```python
from build123d import *

# Parameters (mm, degrees)
SKETCH1_W           = 80
SKETCH1_H           = 80
SKETCH1_R           = 25
BOSS_EXTRUDE1_DEPTH = 10
SKETCH3_W           = 80
SKETCH3_H           = 80
SKETCH3_R           = 25
BOSS_EXTRUDE2_DEPTH = 10
SKETCH4_R           = 25
SKETCH4_W           = 80
SKETCH4_H           = 80
BOSS_EXTRUDE3_DEPTH = 10


with BuildPart() as part:
    # Sketch1 → Boss-Extrude1 (new body)
    with BuildSketch(Plane(origin=(0, 0, 0), x_dir=(1, 0, 0), z_dir=(0, 1, 0))):
        with Locations((40, -40)):
            Rectangle(SKETCH1_W, SKETCH1_H)
        with Locations((40, -40)):
            Circle(SKETCH1_R, mode=Mode.SUBTRACT)
        with Locations((120, -40)):
            Rectangle(SKETCH1_W, SKETCH1_H)
        with Locations((120, -40)):
            Circle(SKETCH1_R, mode=Mode.SUBTRACT)
        with Locations((200, -40)):
            Rectangle(SKETCH1_W, SKETCH1_H)
        with Locations((200, -40)):
            Circle(SKETCH1_R, mode=Mode.SUBTRACT)
        with Locations((200, 40)):
            Rectangle(SKETCH1_W, SKETCH1_H)
        with Locations((200, 40)):
            Circle(SKETCH1_R, mode=Mode.SUBTRACT)
        with Locations((120, 40)):
            Rectangle(SKETCH1_W, SKETCH1_H)
        with Locations((120, 40)):
            Circle(SKETCH1_R, mode=Mode.SUBTRACT)
        with Locations((40, 40)):
            Rectangle(SKETCH1_W, SKETCH1_H)
        with Locations((40, 40)):
            Circle(SKETCH1_R, mode=Mode.SUBTRACT)
        with Locations((40, 120)):
            Rectangle(SKETCH1_W, SKETCH1_H)
        with Locations((40, 120)):
            Circle(SKETCH1_R, mode=Mode.SUBTRACT)
        with Locations((120, 120)):
            Rectangle(SKETCH1_W, SKETCH1_H)
        with Locations((120, 120)):
            Circle(SKETCH1_R, mode=Mode.SUBTRACT)
        with Locations((200, 120)):
            Rectangle(SKETCH1_W, SKETCH1_H)
        with Locations((201.671071705, 120)):
            Circle(SKETCH1_R, mode=Mode.SUBTRACT)
    extrude(amount=BOSS_EXTRUDE1_DEPTH)

    # Sketch3 → Boss-Extrude2 (add)
    with BuildSketch(Plane(origin=(0, 0, -160), x_dir=(-1, 0, 0), z_dir=(0, 0, -1))):
        with Locations((-200, 130)):
            Rectangle(SKETCH3_W, SKETCH3_H)
        with Locations((-200, 130)):
            Circle(SKETCH3_R, mode=Mode.SUBTRACT)
        Polygon((-213.333333333, 90), (-240, 90), (-240, 63.333333333), (-240, 36.666666667), (-240, 10), (-213.333333333, 10), (-186.666666667, 10), (-160, 10), (-160, 36.666666667), (-160, 63.333333333), (-160, 90), (-186.666666667, 90), align=None)
        with Locations((-200, 50)):
            Circle(SKETCH3_R, mode=Mode.SUBTRACT)
        Polygon((-213.333333333, 10), (-240, 10), (-240, 0), (0, 0), (0, 10), (-26.666666667, 10), (-53.333333333, 10), (-80, 10), (-106.666666667, 10), (-133.333333333, 10), (-160, 10), (-186.666666667, 10), align=None)
        Polygon((-133.333333333, 90), (-160, 90), (-160, 63.333333333), (-160, 36.666666667), (-160, 10), (-133.333333333, 10), (-106.666666667, 10), (-80, 10), (-80, 36.666666667), (-80, 63.333333333), (-80, 90), (-106.666666667, 90), align=None)
        with Locations((-120, 50)):
            Circle(SKETCH3_R, mode=Mode.SUBTRACT)
        Polygon((-53.333333333, 90), (-80, 90), (-80, 63.333333333), (-80, 36.666666667), (-80, 10), (-53.333333333, 10), (-26.666666667, 10), (0, 10), (0, 36.666666667), (0, 63.333333333), (0, 90), (-26.666666667, 90), align=None)
        with Locations((-40, 50)):
            Circle(SKETCH3_R, mode=Mode.SUBTRACT)
        with Locations((-40, 130)):
            Rectangle(SKETCH3_W, SKETCH3_H)
        with Locations((-40, 130)):
            Circle(SKETCH3_R, mode=Mode.SUBTRACT)
        with Locations((-120, 130)):
            Rectangle(SKETCH3_W, SKETCH3_H)
        with Locations((-120, 130)):
            Circle(SKETCH3_R, mode=Mode.SUBTRACT)
        with Locations((-120, 210)):
            Rectangle(SKETCH3_W, SKETCH3_H)
        with Locations((-120, 210)):
            Circle(SKETCH3_R, mode=Mode.SUBTRACT)
        with Locations((-40, 210)):
            Rectangle(SKETCH3_W, SKETCH3_H)
        with Locations((-40, 210)):
            Circle(SKETCH3_R, mode=Mode.SUBTRACT)
        with Locations((-200, 210)):
            Rectangle(SKETCH3_W, SKETCH3_H)
        with Locations((-200, 210)):
            Circle(SKETCH3_R, mode=Mode.SUBTRACT)
    extrude(amount=BOSS_EXTRUDE2_DEPTH)

    # Sketch4 → Boss-Extrude3 (add)
    with BuildSketch(Plane.ZY):
        Polygon((-133.333333333, 90), (-160, 90), (-160, 63.333333333), (-160, 36.666666667), (-160, 10), (-133.333333333, 10), (-106.666666667, 10), (-80, 10), (-80, 36.666666667), (-80, 63.333333333), (-80, 90), (-106.666666667, 90), align=None)
        with Locations((-120, 50)):
            Circle(SKETCH4_R, mode=Mode.SUBTRACT)
        Polygon((-133.333333333, 170), (-160, 170), (-160, 143.333333333), (-160, 116.666666667), (-160, 90), (-133.333333333, 90), (-106.666666667, 90), (-80, 90), (-80, 116.666666667), (-80, 143.333333333), (-80, 170), (-106.666666667, 170), align=None)
        with Locations((-120, 130)):
            Circle(SKETCH4_R, mode=Mode.SUBTRACT)
        Polygon((-160, 196.666666667), (-160, 170), (-133.333333333, 170), (-106.666666667, 170), (-80, 170), (-80, 196.666666667), (-80, 223.333333333), (-80, 250), (-106.666666667, 250), (-133.333333333, 250), (-160, 250), (-160, 223.333333333), align=None)
        with Locations((-120, 210)):
            Circle(SKETCH4_R, mode=Mode.SUBTRACT)
        with Locations((-40, 210)):
            Rectangle(SKETCH4_W, SKETCH4_H)
        with Locations((-40, 210)):
            Circle(SKETCH4_R, mode=Mode.SUBTRACT)
        with Locations((-40, 130)):
            Rectangle(SKETCH4_W, SKETCH4_H)
        with Locations((-40, 130)):
            Circle(SKETCH4_R, mode=Mode.SUBTRACT)
        Polygon((-53.333333333, 90), (-80, 90), (-80, 63.333333333), (-80, 36.666666667), (-80, 10), (-53.333333333, 10), (-26.666666667, 10), (0, 10), (0, 36.666666667), (0, 63.333333333), (0, 90), (-26.666666667, 90), align=None)
        with Locations((-40, 50)):
            Circle(SKETCH4_R, mode=Mode.SUBTRACT)
        Polygon((53.333333333, 10), (80, 10), (80, 36.666666667), (80, 63.333333333), (80, 90), (53.333333333, 90), (26.666666667, 90), (0, 90), (0, 63.333333333), (0, 36.666666667), (0, 10), (26.666666667, 10), align=None)
        with Locations((40, 50)):
            Circle(SKETCH4_R, mode=Mode.SUBTRACT)
        with Locations((40, 130)):
            Rectangle(SKETCH4_W, SKETCH4_H)
        with Locations((40, 130)):
            Circle(SKETCH4_R, mode=Mode.SUBTRACT)
        with Locations((40, 210)):
            Rectangle(SKETCH4_W, SKETCH4_H)
        with Locations((40, 210)):
            Circle(SKETCH4_R, mode=Mode.SUBTRACT)
        Polygon((-160, 143.333333333), (-160, 170), (-160, 196.666666667), (-160, 223.333333333), (-160, 250), (-170, 250), (-170, 0), (80, 0), (80, 10), (53.333333333, 10), (26.666666667, 10), (0, 10), (-26.666666667, 10), (-53.333333333, 10), (-80, 10), (-106.666666667, 10), (-133.333333333, 10), (-160, 10), (-160, 36.666666667), (-160, 63.333333333), (-160, 90), (-160, 116.666666667), align=None)
    extrude(amount=BOSS_EXTRUDE3_DEPTH)


solid = part.part
```
CAD build for the part. Positions are in the model's coordinates, mm. A direction names the side the tool comes from. Give positions to 0.01 mm unless a question says otherwise; leave off trailing zeros. Write each loop counter-clockwise with the first axis right and the second up, starting at its lowest first coordinate (ties: lowest second). Pieces come first, ordered by that corner, then holes. Notation, with made-up numbers: M 2,-37.5 L 20,-37.5 A14 ccw 20,-12.5 Z; hole C 81,30.25 d2. An arc over 180 degrees is marked long. Return JSON: item names as keys, results as strings. Group by question number.
(1) Band-saw the part on C-C (y = 97). Give the cut face in (x, z), and give its area (3 significant figures).
(2) Band-saw the part on A-A (x = 120). State how many separate pieces and enclosed holes the cut face has, and give its area (3 significant figures).
(3) Band-saw the part on D-D (x = 71.5). Give the cut face in (y, z), and give its area (3 significant figures).
(4) Mould opens along X. For faces 3 (the face through (0, 132, -68)), 4 (the face through (60, 250, -165)), 5 (the face through (176.91, 40.42, -164.93)) say: pulls with the +X half, pulls with the -X half, needs draft (parallel to the pull), parting line crosses it, or undercut.
(5) Drill centre lines: L1, parallel to Y at x = -2.75, z = -120; L2, parallel to X at y = 3.25, z = 40; L3, parallel to X at y = 3, z = -120. Where is each one in solid material? Low to high. Write a range as [from, to].
(6) 3-axis set-ups, long thin cutter, end or side, ignore diameter. For faces 1 (the face through (-4.93, 234.787, -43.255)), 2 (the face through (92, 10, -42)): which of +Z, -Z, +X, -X, +Y, -Y reach the whole face in a straight line?
(7) Flat gauge pins, fed straight in: pin 1 Ø2 at (x, z) = (38.5, -89) entering from +Y; pin 2 Ø10 at (x, y) = (209.5, 63.5) entering from -Z. Where does each tip first touch, or does it go through?
Entries:
{
 "1": {"outline": "M -10,-170 L 240,-170 L 240,-160 L 0,-160 L 0,80 L -10,80 Z", "area": "4,900 mm^2"},
 "2": {"separate pieces": "7", "enclosed holes": "0", "area": "1,900 mm^2"},
 "3": {"outline": "M 0,-170 L 250,-170 L 250,-160 L 10,-160 L 10,80 L 0,80 Z", "area": "4,900 mm^2"},
 "4": {"face 3": "pulls with the +X half", "face 4": "needs draft", "face 5": "undercut"},
 "5": {"L1": "y = [0, 25], [75, 105], [155, 185], [235, 250]", "L2": "x = [-10, 15], [65, 95], [145, 175], [225, 240]", "L3": "x = [-10, 15], [65, 95], [145, 176.67], [226.67, 240]"},
 "6": {"face 1": "+X, -X", "face 2": "+Z, +X, +Y"},
 "7": {"pin 1": "stops at y = 10", "pin 2": "passes through"}
}
